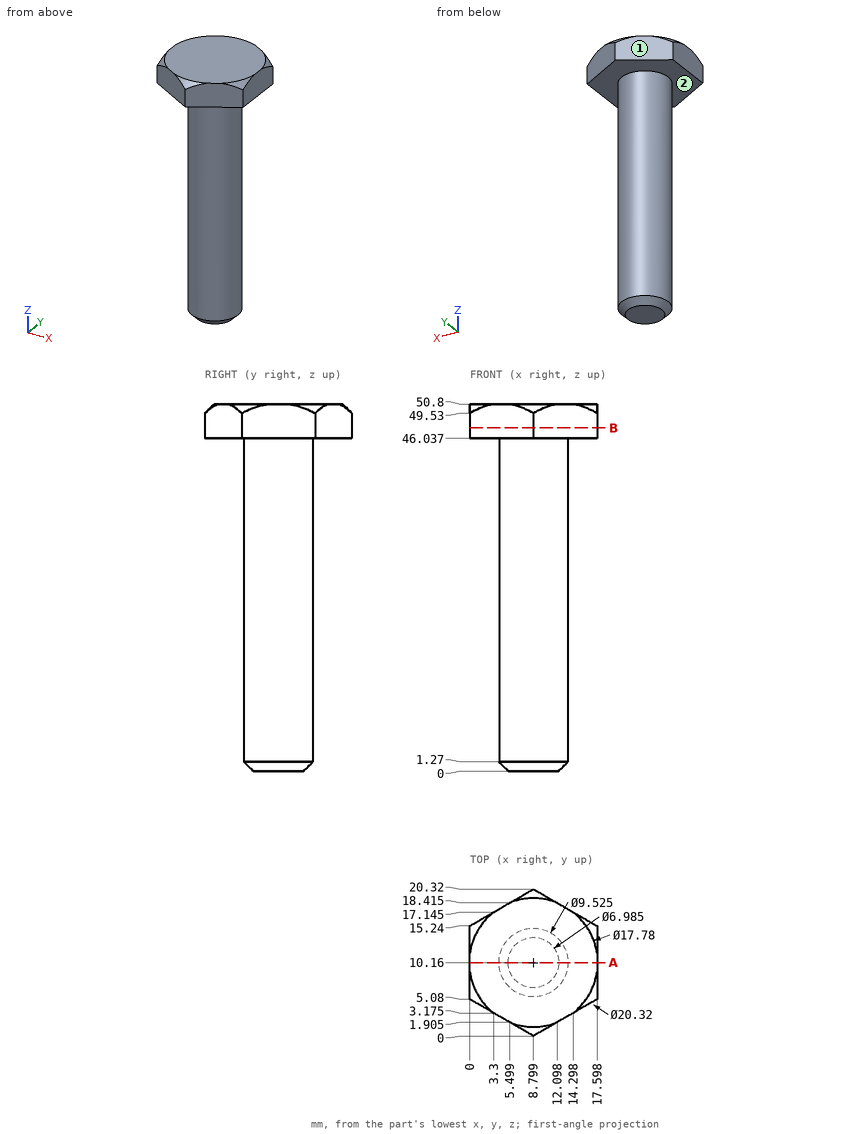
The drawing under review shows one solid part. Ordinate dimensions are in mm from its lowest x, y, z. A direction names the side the tool comes from. Give positions to 0.01 mm unless a question says otherwise; leave off trailing zeros. Write each loop counter-clockwise with the first axis right and the second up, starting at its lowest first coordinate (ties: lowest second). Pieces come first, ordered by that corner, then holes.
1. Add section B-B, the plane z = 47.5. Write out the cut boundary in (x, y), plus the area to 3 significant figures.
2. Wall thickness on L1, parallel to Z at x = 2, y = 7; L2, parallel to X at y = 7.75, z = 27 (1 decimal); L3, parallel to Y at x = 8.75, z = 19.5: over which ranges is each line inside the solid? List them lowest first.
3. Tool access review of the marked faces 1 and 2: name each direction out of +Z, -Z, +X, -X, +Y, -Y from which nothing blocks a thin tool from reaching the whole face with its end or side.
4. Add section A-A, the plane y = 10.16. Write out the cut boundary in (x, z), plus the area to 3 significant figures.
5. For P1, Ø12, axis at y = 7.5, z = 38, coming from the +X side; P2, Ø4, axis at y = 4.5, z = 44, coming from the +X side (1 decimal); P3, Ø2, axis at x = 10, y = 2, coming from the -Z side, all flat-tipped, find the tip position at first contact; note any pin that passes through.
Worked answers:
1. outline: (0, 5.08) - (8.8, 0) - (17.6, 5.08) - (17.6, 15.24) - (8.8, 20.32) - (0, 15.24) - close
1. area: 268 mm2
2. L1: z = 46.04 to 50.8
2. L2: x = 4.7 to 12.9
2. L3: y = 5.4 to 14.92
3. face 1: +Z, -Z, -X, +Y
3. face 2: -Z
4. outline: (0, 46.04) - (4.04, 46.04) - (4.04, 1.27) - (5.31, 0) - (12.29, 0) - (13.56, 1.27) - (13.56, 46.04) - (17.6, 46.04) - (17.6, 50.8) - (0, 50.8) - close
4. area: 521 mm2
5. P1: stops at x = 13.56
5. P2: stops at x = 11.8
5. P3: stops at z = 46.04
